```python
from build123d import *

# Parameters (mm, degrees)
SKETCH_1_R      = 3.5
SKETCH_1_R_2    = 1.5
EXTRUDE_1_DEPTH = 6.5


with BuildPart() as part:
    # 草图1 → 凸台-拉伸1 (new body)
    with BuildSketch(Plane(origin=(0, 0, 0), x_dir=(1, 0, 0), z_dir=(0, 1, 0))):
        with Locations(Location((0, 0, 0), (0, 0, 90))):
            Circle(SKETCH_1_R)
        with Locations(Location((0, 0, 0), (0, 0, 90))):
            Circle(SKETCH_1_R_2, mode=Mode.SUBTRACT)
    extrude(amount=EXTRUDE_1_DEPTH)

    # 草图3 → 旋转5 (revolve)
    with BuildSketch(Plane(origin=(0, 4.5, 0), x_dir=(1, 0, 0), z_dir=(0, 1, 0))):
        with BuildLine():
            Line((-1.55, 0), (1.55, 0))
            ThreePointArc((1.55, 0), (0, -1.55), (-1.55, 0))
        make_face()
    revolve(axis=Axis((-3.959014724, 4.5, 0), (1, 0, 0)))


solid = part.part
```
Read the model definition and answer for the solid it produces. Units are mm, in the model's axes. Give positions to 0.01 mm unless a question says otherwise; leave off trailing zeros. Order: outer loops, then holes, each group sorted by start corner. A loop starts at its lowest first (then second) coordinate and runs counter-clockwise, first axis right, second up.
(1) Find section B-B (z = 0). Give the vertices of the cut face in (x, y).
(2) Straight lines are drawn through the part: L1, parallel to X at y = 1.45, z = 0; L2, parallel to X at y = 3.75, z = -1; L3, parallel to X at y = 5.85, z = 0. For each, find the intervals that lie inside material, in ascending order.
(3) Given pin 1 (1 mm diameter, centred on x = -1.5, y = 2, fed in from -Z), flat-ended and moving along its own axis, determine where the tip first touches the part or whether it passes through.
(4) Find section A-A (x = 0). Give the vertices of the cut face in (y, z), plus the area to 3 significant figures.
(5) Find section D-D (y = 2). Give the vertices of the cut face in (x, z), plus the area to 3 significant figures.
(6) Find section C-C (y = 5). Give the vertices of the cut face in (x, z).
(7) For a pull along X with two mould halves and no side action, classify faces 1 (the flat face through (0, 6.5, -2)), 2 (the cylindrical face through (-0.45, 2.03, -1.43)), 3 (the cylindrical face through (3.417, 3.204, 0.759)) as released by +X, released by -X, zero draft, split by the parting line, or undercut.
Result sheet:
1. outline: (-3.5, 0) - (-1.5, 0) - (-1.5, 4.11) arc R1.55 ccw to (1.5, 4.11) - (1.5, 0) - (3.5, 0) - (3.5, 6.5) - (1.5, 6.5) - (1.5, 4.89) arc R1.55 ccw to (-1.5, 4.89) - (-1.5, 6.5) - (-3.5, 6.5) - close
2. L1: x = -3.5 to -1.5, 1.5 to 3.5
2. L2: x = -3.35 to -1.12, -0.92 to 0.92, 1.12 to 3.35
2. L3: x = -3.5 to -1.5, -0.76 to 0.76, 1.5 to 3.5
3. pin 1: stops at z = -3.35
4. outline: (0, -3.5) - (6.5, -3.5) - (6.5, -1.5) - (4.89, -1.5) arc R1.55 ccw to (4.89, 1.5) - (6.5, 1.5) - (6.5, 3.5) - (0, 3.5) - (0, 1.5) - (4.11, 1.5) arc R1.55 ccw to (4.11, -1.5) - (0, -1.5) - close
4. area: 33.5 mm2
5. outline: circle Ø7 at (0, 0); hole circle Ø3 at (0, 0)
5. area: 31.4 mm2
6. outline: circle Ø7 at (0, 0); circle Ø2.93 at (0, 0); hole circle Ø3 at (0, 0)
7. face 1: zero draft
7. face 2: undercut
7. face 3: split by the parting line
